Autodesk Inventor part; units mm, degrees
ref_plane "YZ Plane" through (0, 0, 0) normal (1, 0, 0) x (0, 1, 0)
ref_plane "XZ Plane" through (0, 0, 0) normal (0, 1, 0) x (-1, 0, 0)
ref_plane "XY Plane" through (0, 0, 0) normal (0, 0, 1) x (1, 0, 0)
sketch "スケッチ1" plane through (0, 0, 0) normal (0, 0, 1) x (1, 0, 0)
  circle A0 centre (0, 0) radius 22.5
  dimension "d0" = 45
extrude "押し出し1" add sketch "スケッチ1" along normal blind 53.5
sketch "スケッチ2" plane through (0, 0, 53.5) normal (0, 0, 1) x (1, 0, 0)
  circle A0 centre (0, 0) radius 7.5
  dimension "d3" = 15
extrude "押し出し2" add sketch "スケッチ2" along normal blind 4.3
sketch "スケッチ3" plane through (0, 0, 0) normal (0, 0, -1) x (-1, 0, 0)
  circle A0 centre (0, 0) radius 7.5
  circle A1 centre (0, 0) radius 14.5
  point P0 (0, 14.5)
  point P1 (0, -14.5)
  dimension "d6" = 29
hole "穴1" at (0, 14.5, 0) at (0, -14.5, 0) direction (0, 0, 1) diameter 4 depth 4 tip angle 118
sketch "スケッチ4" plane through (0, 0, 0) normal (0, 0, -1) x (-1, 0, 0)
  circle A0 centre (0, 0) radius 7.5
  circle A1 centre (0, 0) radius 2.5
  dimension "d14" = 15
  dimension "d15" = 5
extrude "押し出し3" add sketch "スケッチ4" along normal blind 11.9 contours A1
sketch "スケッチ5" plane through (0, 0, 0) normal (0, 0, -1) x (-1, 0, 0)
  circle A0 centre (0, 0) radius 2.5
  circle A1 centre (0, 0) radius 7.5
  dimension "d18" = 15
extrude "押し出し4" add sketch "スケッチ5" along normal blind 4.4
properties part number "rz735"
Geometry: final body of the model. Coordinates: model frame, mm. A direction names the side the tool comes from. Give positions to 0.01 mm unless a question says otherwise; leave off trailing zeros. Order: outer loops, then holes, each group sorted by start corner. A loop starts at its lowest first (then second) coordinate and runs counter-clockwise, first axis right, second up. Notation, with made-up numbers: (88, -17) -> (146, -17) arc R10 cw to (146, 1) -> close; hole circle Ø1 at (-8.75, 63). An arc over 180 degrees is marked (long way). Write each question's results on one line, items separated by ' | '. Start each with the question number.
1) Set-up query: faces 1 (the cylindrical face through (7.493, -0.33, -2.169)), 2 (the flat face through (0, 0, 57.8)), 3 (the flat face through (0, -10, 53.5)). Return all of +Z, -Z, +X, -X, +Y, -Y with unobstructed straight access to the full face (end or side cutting, diameter ignored); none if empty.
2) Section D-D (y = -5). Return loops of the section in (x, z).
3) Draft query along X for faces 4 (the cylindrical face through (1.2, -16.1, 2)), 5 (the flat face through (0, -10, 0)), 6 (the cylindrical face through (10.382, 19.961, 26.376)). Return one class per face: pulls with the +X half, pulls with the -X half, needs draft (parallel to the pull), parting line crosses it, or undercut.
4) Section A-A (y = 0). Return loops of the section in (x, z).
5) Section C-C (z = 47). Return loops of the section in (x, y), then the cut area to 3 significant figures.
6) Line query: line 1 (Y direction, x = 0, z = 3.2); line 2 (Z direction, x = 0, y = -8); line 3 (X direction, y = -14, z = 1). Output: solid intervals per line, ascending. Write a range as from..to.
7) First-contact query: pin 1 (5 mm diameter, centred on y = 8.5, z = 50.5, fed in from +X); pin 2 (3 mm diameter, centred on x = 0, y = -14.5, fed in from -Z); pin 3 (1.5 mm diameter, centred on x = -14, z = 22, fed in from +Y). Flat tips, straight axial feed; report the tip coordinate or a pass-through.
8) Section B-B (x = -18). Return loops of the section in (y, z), then the cut area to 3 significant figures.
Calculated:
1) face 1: -Z | face 2: +Z, +X, -X, +Y, -Y | face 3: +Z
2) outline: (-21.94, 0) -> (-5.59, 0) -> (-5.59, -4.4) -> (5.59, -4.4) -> (5.59, 0) -> (21.94, 0) -> (21.94, 53.5) -> (5.59, 53.5) -> (5.59, 57.8) -> (-5.59, 57.8) -> (-5.59, 53.5) -> (-21.94, 53.5) -> close
3) face 4: undercut | face 5: needs draft | face 6: parting line crosses it
4) outline: (-22.5, 0) -> (-7.5, 0) -> (-7.5, -4.4) -> (-2.5, -4.4) -> (-2.5, -11.9) -> (2.5, -11.9) -> (2.5, -4.4) -> (7.5, -4.4) -> (7.5, 0) -> (22.5, 0) -> (22.5, 53.5) -> (7.5, 53.5) -> (7.5, 57.8) -> (-7.5, 57.8) -> (-7.5, 53.5) -> (-22.5, 53.5) -> close
5) outline: circle Ø45 at (0, 0) | area: 1,590 mm2
6) line 1: -22.5..-16.5, -12.5..12.5, 16.5..22.5 | line 2: 0..53.5 | line 3: -17.61..-1.94, 1.94..17.61
7) pin 1: x = 21.69 | pin 2: z = 4.3 | pin 3: y = 18.18
8) outline: (-13.5, 0) -> (13.5, 0) -> (13.5, 53.5) -> (-13.5, 53.5) -> close | area: 1,440 mm2
